Verification items for this drawing (mm, ordinates from the low corner). A direction names the side the tool comes from. Round coordinates to 2 decimals unless told otherwise and drop trailing zeros. Write each loop counter-clockwise with the first axis right and the second up, starting at its lowest first coordinate (ties: lowest second). Pieces come first, ordered by that corner, then holes. Notation, with made-up numbers: M 75,-2 L 89,-2 A26 cw 89,14 Z; hole C -7.75,40.25 d9. An arc over 180 degrees is marked long. One line per question, with ' | ' between items. Start each with the question number.
Q1. Cross-section at D-D (z = 8.5). Record the boundary of the cut face in (x, y).
Q2. Thickness scan on line 1 along Z through (x, y) = (4, 12.7) (1 decimal); line 2 along Z through (x, y) = (36, 16); line 3 along X through (y, z) = (16.75, 20). Record the ranges inside material, lowest first. Write a range as from..to.
Q3. Tool access check on the marked faces 1 and 2. Record the directions out of +Z, -Z, +X, -X, +Y, -Y that give a thin tool (end or side, any length) a straight path to the whole face; none if there is none.
Q4. Cross-section at B-B (x = 11). Record the boundary of the cut face in (y, z).
Q5. Cross-section at C-C (y = 7.62). Record the boundary of the cut face in (x, z).
Q6. Gauge pin test, flat ends, axial feed: pin 1 (9 mm diameter, centred on x = 12.7, y = 7.62, fed in from +Z); pin 2 (12.5 mm diameter, centred on y = 8, z = 14.5, fed in from +X). Record the tip position at first contact, or that the pin passes through.
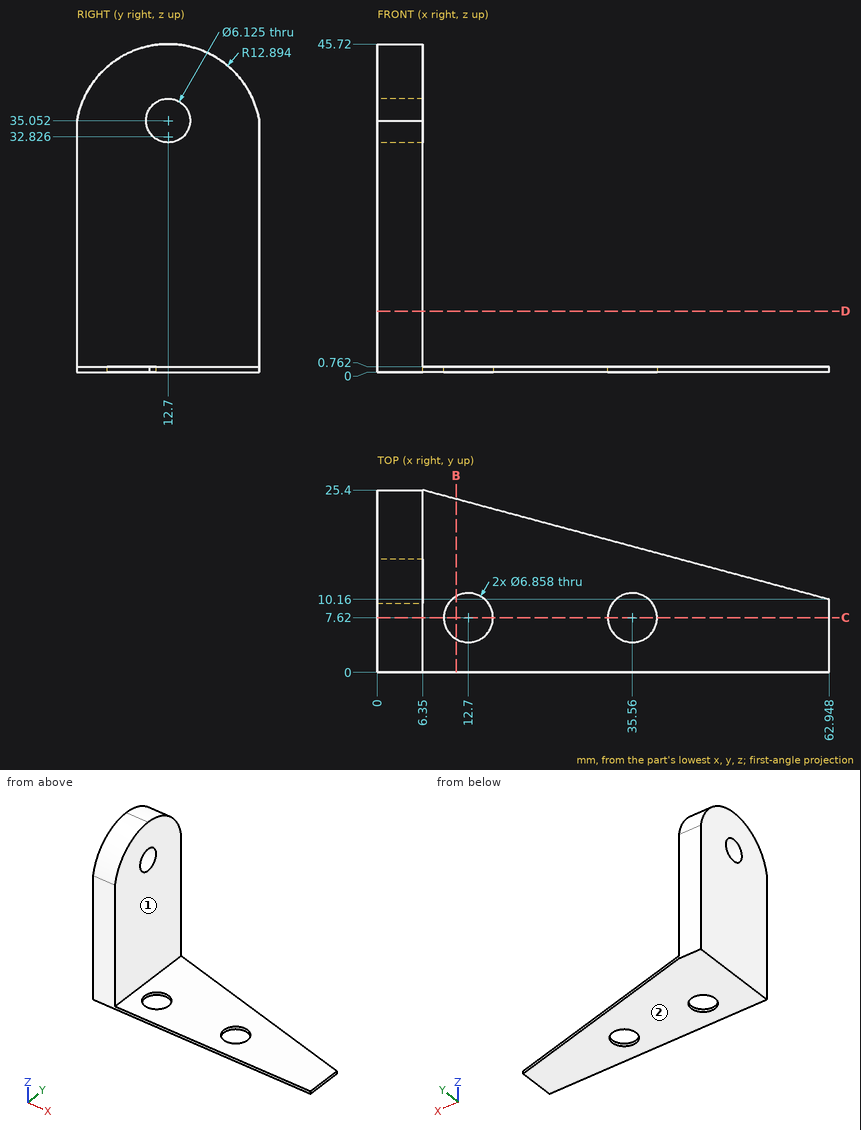
Determined:
1) outline: M 0,0 L 6.35,0 L 6.35,25.4 L 0,25.4 Z
2) line 1: z = 0..32, 38.1..45.7 | line 2: z = 0..0.76 | line 3: x = 0..6.35
3) face 1: +Z, +X, +Y, -Y | face 2: -Z, +X, -X, +Y, -Y
4) outline: M 0,0 L 4.64,0 L 4.64,0.76 L 0,0.76 Z; M 10.6,0 L 24.15,0 L 24.15,0.76 L 10.6,0.76 Z
5) outline: M 0,0 L 9.27,0 L 9.27,0.76 L 6.35,0.76 L 6.35,44.68 L 0,44.68 Z; M 16.13,0 L 32.13,0 L 32.13,0.76 L 16.13,0.76 Z; M 38.99,0 L 62.95,0 L 62.95,0.76 L 38.99,0.76 Z
6) pin 1: stops at z = 0.76 | pin 2: stops at x = 6.35
